Autodesk Inventor part; units mm, degrees
ref_plane "YZ Plane" through (0, 0, 0) normal (1, 0, 0) x (0, 1, 0)
ref_plane "XZ Plane" through (0, 0, 0) normal (0, 1, 0) x (-1, 0, 0)
ref_plane "XY Plane" through (0, 0, 0) normal (0, 0, 1) x (1, 0, 0)
sketch "Skizze1" plane through (0, 0, 0) normal (0, 1, 0) x (-1, 0, 0)
  line L0 (10, 17.6) -> (-10, 17.6)
  line L1 (-10, 17.6) -> (-10, -17.6)
  line L2 (-10, -17.6) -> (10, -17.6)
  line L3 (10, -17.6) -> (10, 17.6)
  line L4 (6.4, 14) -> (-6.4, 14) construction
  line L5 (-6.4, 14) -> (-6.4, -14) construction
  line L6 (-6.4, -14) -> (6.4, -14) construction
  line L7 (6.4, -14) -> (6.4, 14) construction
  line L8 (0, 17.6) -> (0, -17.6) construction
  line L9 (10, 0) -> (-10, 0) construction
  point P0 (0, 0)
  point P1 (0, 0)
  dimension "d0" = 12.8
  dimension "d1" = 28
  dimension "d2" = 20
  dimension "d3" = 3.6
  dimension "d4" = 3.6
extrude "Extrusion1" add sketch "Skizze1" along normal blind 1.5
hole "Bohrung1" at (6.4, 0, 14) direction (0, 1, 0) diameter 1 end through all
pattern_linear "Rechteckige Anordnung1" count 12 spacing 2.5455 along (0, 0, -1) count 6 spacing 2.56 along (-1, 0, 0) of "Bohrung1"
sketch "Skizze2" plane through (0, 0, 0) normal (0, -1, 0) x (1, 0, 0)
  circle A0 centre (6.4, 14) radius 0.5
  circle A1 centre (-6.4, 14) radius 0.5
  circle A2 centre (-6.4, -14) radius 0.5
  circle A3 centre (6.4, -14) radius 0.5
  circle A4 centre (-6.4, -14) radius 0.5
  point P0 (0, 0)
hole "Bohrung2" at (6.4, 0, -14) at (-6.4, 0, -14) at (-6.4, 0, 14) at (6.4, 0, 14) direction (0, 1, 0) diameter 1.6 end through all
equation "\"d4\" = d3"
properties part number "PCB_PowerSupply"
Input: part model. Units: mm. Frame: model coordinates. Give positions to 0.01 mm unless a question says otherwise; leave off trailing zeros. Loops run counter-clockwise (first coordinate to the right, second up) from the corner with the lowest first, then second, coordinate; pieces in that order, holes last. Notation, with made-up numbers: (44.25, 12) -> (91.25, 12) arc R4 ccw to (91.25, 18) -> close; hole circle Ø9 at (68, 34). An arc over 180 degrees is marked (long way). Answer as a JSON object with one key per item and string values. Group by question number.
Item 1: Pull-direction query (X, two-part tool) for faces 1 (the cylindrical face through (-3.648, 0.76, -11.917)), 2 (the flat face through (0, 1, 17.6)), 3 (the flat face through (-10, 1, 0)); classes: released by +X, released by -X, zero draft, split by the parting line, or undercut.
Item 2: Cut plane B-B, the plane x = -6.4. State how many separate pieces and enclosed holes the cut face has, and give its area (3 significant figures).
Item 3: Cut plane A-A, the plane z = -14. Return the cut outline in (x, y), and give its area (3 significant figures).
Item 4: Pin query (flat end, axial travel): P1, Ø1, axis at x = -6.4, z = -14, coming from the -Y side. Return the tip coordinate at first contact, or that it passes through.
Checks:
{
 "1": {"face 1": "undercut", "face 2": "zero draft", "face 3": "released by -X"},
 "2": {"separate pieces": "13", "enclosed holes": "0", "area": "33.0 mm²"},
 "3": {"outline": "(-10, 0) -> (-7.2, 0) -> (-7.2, 1.5) -> (-10, 1.5) -> close; (-5.6, 0) -> (-4.34, 0) -> (-4.34, 1.5) -> (-5.6, 1.5) -> close; (-3.34, 0) -> (-1.78, 0) -> (-1.78, 1.5) -> (-3.34, 1.5) -> close; (-0.78, 0) -> (0.78, 0) -> (0.78, 1.5) -> (-0.78, 1.5) -> close; (1.78, 0) -> (3.34, 0) -> (3.34, 1.5) -> (1.78, 1.5) -> close; (4.34, 0) -> (5.6, 0) -> (5.6, 1.5) -> (4.34, 1.5) -> close; (7.2, 0) -> (10, 0) -> (10, 1.5) -> (7.2, 1.5) -> close", "area": "19.2 mm²"},
 "4": {"P1": "passes through"}
}
